```python
from build123d import *

# Parameters (mm, degrees)
BOSS_EXTRUDE6_DEPTH = 60
SKETCH9_R           = 1.6
CUT_EXTRUDE3_DEPTH  = 50
SKETCH10_R          = 1.15
CUT_EXTRUDE5_DEPTH  = 22.05
SKETCH11_W          = 7
SKETCH11_H          = 60
SKETCH11_R          = 1.6
BOSS_EXTRUDE7_DEPTH = 3
SKETCH12_W          = 7
SKETCH12_H          = 60
SKETCH12_R          = 1.6
BOSS_EXTRUDE8_DEPTH = 3
SKETCH16_R          = 2.5
CUT_EXTRUDE9_DEPTH  = 8.75
SKETCH17_R          = 2.5
CUT_EXTRUDE10_DEPTH = 8.75


with BuildPart() as part:
    # Sketch2 → Boss-Extrude6 (new body)
    with BuildSketch(Plane.XY):
        with BuildLine():
            ThreePointArc((6.475, 0), (0, 6.475), (-6.475, 0))
            Line((-6.475, 0), (-20, 0))
            Line((-20, 0), (-20, 2.847591854))
            Line((-20, 2.847591854), (-13, 2.847591854))
            Line((-13, 2.847591854), (-13, 14.347591854))
            Line((-13, 14.347591854), (13, 14.347591854))
            Line((13, 14.347591854), (13, 2.847591854))
            Line((13, 2.847591854), (20, 2.847591854))
            Line((20, 2.847591854), (20, 0))
            Line((20, 0), (6.475, 0))
        make_face()
    extrude(amount=BOSS_EXTRUDE6_DEPTH)

    # Sketch9 → Cut-Extrude3 (cut)
    with BuildSketch(Plane(origin=(0, 2.847591854, 0), x_dir=(1, 0, 0), z_dir=(0, 1, 0))):
        with Locations((-16.5, -15)):
            Circle(SKETCH9_R)
        with Locations((-16.5, -45)):
            Circle(SKETCH9_R)
        with Locations((16.5, -15)):
            Circle(SKETCH9_R)
        with Locations((16.5, -45)):
            Circle(SKETCH9_R)
    extrude(amount=-CUT_EXTRUDE3_DEPTH, mode=Mode.SUBTRACT)

    # Sketch10 → Cut-Extrude5 (cut)
    with BuildSketch(Plane(origin=(0, 14.347591854, 0), x_dir=(1, 0, 0), z_dir=(0, 1, 0))):
        with Locations((0, -22)):
            Circle(SKETCH10_R)
        with Locations((8, -30)):
            Circle(SKETCH10_R)
        with Locations((-8, -30)):
            Circle(SKETCH10_R)
        with Locations((0, -38)):
            Circle(SKETCH10_R)
    extrude(amount=-CUT_EXTRUDE5_DEPTH, mode=Mode.SUBTRACT)

    # Sketch11 → Boss-Extrude7 (add)
    with BuildSketch(Plane(origin=(0, 2.847591854, 0), x_dir=(1, 0, 0), z_dir=(0, 1, 0))):
        with Locations((16.5, -30)):
            Rectangle(SKETCH11_W, SKETCH11_H)
        with Locations((16.5, -45)):
            Circle(SKETCH11_R, mode=Mode.SUBTRACT)
        with Locations((16.5, -15)):
            Circle(SKETCH11_R, mode=Mode.SUBTRACT)
    extrude(amount=BOSS_EXTRUDE7_DEPTH)

    # Sketch12 → Boss-Extrude8 (add)
    with BuildSketch(Plane(origin=(0, 2.847591854, 0), x_dir=(1, 0, 0), z_dir=(0, 1, 0))):
        with Locations((-16.5, -30)):
            Rectangle(SKETCH12_W, SKETCH12_H)
        with Locations((-16.5, -45)):
            Circle(SKETCH12_R, mode=Mode.SUBTRACT)
        with Locations((-16.5, -15)):
            Circle(SKETCH12_R, mode=Mode.SUBTRACT)
    extrude(amount=BOSS_EXTRUDE8_DEPTH)

    # Sketch16 → Cut-Extrude9 (cut)
    with BuildSketch(Plane(origin=(0, 0, 0), x_dir=(-1, 0, 0), z_dir=(0, -1, 0))):
        with Locations((0, -22)):
            Circle(SKETCH16_R)
        with Locations((0, -38)):
            Circle(SKETCH16_R)
    extrude(amount=-CUT_EXTRUDE9_DEPTH, mode=Mode.SUBTRACT)

    # Sketch17 → Cut-Extrude10 (cut)
    with BuildSketch(Plane(origin=(0, 0, 0), x_dir=(-1, 0, 0), z_dir=(0, -1, 0))):
        with Locations((-8, -30)):
            Circle(SKETCH17_R)
        with Locations((8, -30)):
            Circle(SKETCH17_R)
    extrude(amount=-CUT_EXTRUDE10_DEPTH, mode=Mode.SUBTRACT)


solid = part.part
```
Here's how the part is built. I have some questions about the finished solid (model axes, mm). A direction names the side the tool comes from. Coordinates: 2 decimals unless noted, no trailing zeros. Order: outer loops, then holes, each group sorted by start corner. A loop starts at its lowest first (then second) coordinate and runs counter-clockwise, first axis right, second up.
Item 1: I'm going to push flat-ended pins straight in: pin 1 Ø3 at (x, z) = (0, 22) entering from -Y; pin 2 Ø1.4 at (x, z) = (8, 30) entering from -Y; pin 3 Ø1.5 at (x, y) = (-2.5, 10) entering from -Z; pin 4 Ø5 at (x, z) = (16.5, 15) entering from +Y. Where does each tip first touch, or does it pass through?
Response values:
pin 1: stops at y = 8.75
pin 2: passes through
pin 3: stops at z = 0
pin 4: stops at y = 5.85
Item 2: Thinking about a two-plate mould opening in Z: for faces 1 (the face through (0, 7, 60)), 2 (the face through (-13, 0, 30)), 3 (the face through (-2.385, 7.34, 21.249)), 4 (the face through (-1, 8.75, 39)), which applies, pulls with the +Z half, pulls with the -Z half, needs draft (parallel to the pull), parting line crosses it, or undercut?
Response values:
face 1: pulls with the +Z half
face 2: needs draft
face 3: undercut
face 4: undercut
Item 3: If we section it at A-A, the plane z = 45: List the corners of the cut face in (x, y) for me (3 decimals).
Response values:
outline: (-20, 0) - (-18.1, 0) - (-18.1, 5.848) - (-20, 5.848) - close; (-14.9, 0) - (-6.475, 0) arc R6.475 cw to (6.475, 0) - (14.9, 0) - (14.9, 5.848) - (13, 5.848) - (13, 14.348) - (-13, 14.348) - (-13, 5.848) - (-14.9, 5.848) - close; (18.1, 0) - (20, 0) - (20, 5.848) - (18.1, 5.848) - close
Item 4: If we section it at D-D, the plane y = 11.5: List the corners of the cut face in (x, z) for me.
Response values:
outline: (-13, 0) - (13, 0) - (13, 60) - (-13, 60) - close; hole circle Ø2.3 at (-8, 30); hole circle Ø2.3 at (0, 22); hole circle Ø2.3 at (0, 38); hole circle Ø2.3 at (8, 30)
Item 5: I need wall thicknesses on probe 1 along Z at (x, y) = (0, 6.7); probe 2 along Z at (x, y) = (16.5, 4.05); probe 3 along X at (y, z) = (10, 38). Which ranges of each line are inside material? Lowest first, please.
Response values:
probe 1: z = 0 to 19.5, 24.5 to 35.5, 40.5 to 60
probe 2: z = 0 to 13.4, 16.6 to 43.4, 46.6 to 60
probe 3: x = -13 to -1.15, 1.15 to 13
Item 6: If we section it at B-B, the plane x = 0: List the corners of the cut face in (y, z) for me (3 decimals).
Response values:
outline: (6.475, 0) - (14.348, 0) - (14.348, 20.85) - (8.75, 20.85) - (8.75, 19.5) - (6.475, 19.5) - close; (6.475, 24.5) - (8.75, 24.5) - (8.75, 23.15) - (14.348, 23.15) - (14.348, 36.85) - (8.75, 36.85) - (8.75, 35.5) - (6.475, 35.5) - close; (6.475, 40.5) - (8.75, 40.5) - (8.75, 39.15) - (14.348, 39.15) - (14.348, 60) - (6.475, 60) - close
Item 7: If we section it at C-C, the plane z = 22: List the corners of the cut face in (x, y) for me (3 decimals).
Response values:
outline: (-20, 0) - (-6.475, 0) arc R6.475 cw to (-2.5, 5.973) - (-2.5, 8.75) - (-1.15, 8.75) - (-1.15, 14.348) - (-13, 14.348) - (-13, 5.848) - (-20, 5.848) - close; (1.15, 8.75) - (2.5, 8.75) - (2.5, 5.973) arc R6.475 cw to (6.475, 0) - (20, 0) - (20, 5.848) - (13, 5.848) - (13, 14.348) - (1.15, 14.348) - close
Item 8: Which directions (+Z, -Z, +X, -X, +Y, -Y) give clear straight access to the entire face, cutting with the end or side of a thin tool? Please do faces 5 (the face through (0, 7, 0)), 6 (the face through (-17, 5.848, 30)), 7 (the face through (13, 10, 30)), 8 (the face through (7, 8.75, 31)).
Response values:
face 5: -Z, +X, -X, +Y, -Y
face 6: +Z, -Z, -X, +Y
face 7: +Z, -Z, +X, +Y
face 8: -Y
